Autodesk Fusion 360 part; units mm, degrees
sketch "Sketch1" plane through (0, 0, 0) normal (0, 0, 1) x (1, 0, 0)
  line L0 (0, 0) -> (50, 0)
  line L1 (50, 0) -> (50, 50)
  line L2 (50, 50) -> (0, 50)
  line L3 (0, 50) -> (0, 0)
  dimension "d3" = 50
  dimension "d4" = 50
extrude "Extrude1" add sketch "Sketch1" along normal blind 2.5
sketch "Sketch2" plane through (0, 0, 2.5) normal (0, 0, 1) x (-1, 0, 0)
  line L0 (0, -50) -> (0, 0)
  line L1 (0, 0) -> (-50, 0)
  line L2 (-50, 0) -> (-50, -50)
  line L3 (-50, -50) -> (0, -50)
  line L4 (0, -25) -> (-50, -25)
  line L5 (0, -26) -> (-50, -26)
  line L6 (-50, -26) -> (-50, -24)
  line L7 (-50, -24) -> (0, -24)
  line L8 (0, -24) -> (0, -26)
  dimension "d5" = 1
  dimension "d6" = 1
extrude "Extrude2" add sketch "Sketch2" along normal blind 80 contours L0 L2 L4 L5 L6 L8 | L0 L2 L4 L6 L7 L8
fillet "Fillet1" radius 7.5 2 edges at (25, 24, 2.5) (25, 26, 2.5)
sketch "Sketch3" plane through (0, 24, 0) normal (0, -1, 0) x (1, 0, 0)
  line L0 (0, 10) -> (50, 10)
  line L1 (50, 10) -> (50, 82.5)
  line L2 (50, 82.5) -> (0, 82.5)
  line L3 (0, 82.5) -> (0, 10)
  line L4 (0, 46.25) -> (50, 46.25)
  line L5 (25, 82.5) -> (25, 0)
  circle A0 centre (25, 56.75) radius 1.5
  circle A1 centre (14.5, 46.25) radius 1.5
  circle A2 centre (35.5, 46.25) radius 1.5
  circle A3 centre (25, 35.75) radius 1.5
  dimension "d11" = 3
  dimension "d12" = 10.5
  dimension "d13" = 3
  dimension "d14" = 10.5
extrude "Extrude3" cut sketch "Sketch3" against normal blind 3 contours L5 A3 | L5 A3 | L4 A1 | L4 A1 | L4 A2 | L4 A2 | L5 A0 | L5 A0
Model file for the job. Use its own axes, mm. A direction names the side the tool comes from. Give positions to 0.01 mm unless a question says otherwise; leave off trailing zeros. Loops run counter-clockwise (first coordinate to the right, second up) from the corner with the lowest first, then second, coordinate; pieces in that order, holes last.
Item 1: Mould opens along Z. For faces 1 (the face through (25, 25, 0)), 2 (the face through (14.175, 24.986, 44.786)), 3 (the face through (24.65, 21.861, 4.755)), 4 (the face through (0, 25, 20)) say: +Z half, -Z half, draft (parallel to the pull), parting line (faces both ways), or undercut.
Check values:
face 1: -Z half
face 2: undercut
face 3: +Z half
face 4: draft
Item 2: Slice it at A-A (z = 46.25). Write the cut outline in (x, y), plus the area to 3 significant figures.
Check values:
outline: (0, 24) - (13, 24) - (13, 26) - (0, 26) - close; (16, 24) - (34, 24) - (34, 26) - (16, 26) - close; (37, 24) - (50, 24) - (50, 26) - (37, 26) - close
area: 88.0 mm2
Item 3: Slice it at B-B (x = 25). Write the cut outline in (y, z).
Check values:
outline: (0, 0) - (50, 0) - (50, 2.5) - (33.5, 2.5) arc R7.5 cw to (26, 10) - (26, 34.25) - (24, 34.25) - (24, 10) arc R7.5 cw to (16.5, 2.5) - (0, 2.5) - close; (24, 37.25) - (26, 37.25) - (26, 55.25) - (24, 55.25) - close; (24, 58.25) - (26, 58.25) - (26, 82.5) - (24, 82.5) - close
Item 4: Which spindle directions (+Z, -Z, +X, -X, +Y, -Y) get a long thin tool onto all of the face, cutting with end or side? Do faces 5 (the face through (25, 24, 46)), 6 (the face through (25, 26, 46)), 7 (the face through (23.81, 24.99, 34.84)). Say none if no direction does.
Check values:
face 5: +Z, +X, -X, -Y
face 6: +Z, +X, -X, +Y
face 7: +Y, -Y
Item 5: Drill centre lines: line 1 along Z through (x, y) = (25, 25); line 2 along Z through (x, y) = (14.5, 24.85); line 3 along X through (y, z) = (25.15, 56.75). Where is each one in solid material? Low to high.
Check values:
line 1: z = 0 to 34.25, 37.25 to 55.25, 58.25 to 82.5
line 2: z = 0 to 44.75, 47.75 to 82.5
line 3: x = 0 to 23.5, 26.5 to 50
Item 6: Drop flat-ended pins along their axis: P1, Ø5, axis at x = 35.5, z = 46.25, coming from the -Y side; P2, Ø12, axis at x = 32.5, z = 14.5, coming from the +Y side; P3, Ø5, axis at x = 36, y = 43.5, coming from the +Z side; P4, Ø2, axis at x = 21, y = 10.5, coming from the -Z side. Give the stop position or say it passes through.
Check values:
P1: stops at y = 24
P2: stops at y = 26.15
P3: stops at z = 2.5
P4: stops at z = 0
Item 7: Slice it at C-C (x = 35.5). Write the cut outline in (y, z), plus the area to 3 significant figures.
Check values:
outline: (0, 0) - (50, 0) - (50, 2.5) - (33.5, 2.5) arc R7.5 cw to (26, 10) - (26, 44.75) - (24, 44.75) - (24, 10) arc R7.5 cw to (16.5, 2.5) - (0, 2.5) - close; (24, 47.75) - (26, 47.75) - (26, 82.5) - (24, 82.5) - close
area: 303 mm2
Item 8: Slice it at D-D (z = 56.75). Write the cut outline in (x, y).
Check values:
outline: (0, 24) - (23.5, 24) - (23.5, 26) - (0, 26) - close; (26.5, 24) - (50, 24) - (50, 26) - (26.5, 26) - close
